Source: CAD feature listing. Evaluate the final solid. Frame: model axes, mm. A direction names the side the tool comes from. Round coordinates to 2 decimals unless told otherwise and drop trailing zeros. Write each loop counter-clockwise with the first axis right and the second up, starting at its lowest first coordinate (ties: lowest second). Pieces come first, ordered by that corner, then holes. Notation, with made-up numbers: (-21.5, 36) - (10.5, 36) arc R12 ccw to (10.5, 58) - close; hole circle Ø9 at (-20, 47). An arc over 180 degrees is marked (long way). Write item = value, one per line. Start each with the question number.
```python
from build123d import *

# Parameters (mm, degrees)
F1_DEPTH = 30
F2_W     = 40
F2_H     = 30
F3_DEPTH = 30
F5_DEPTH = 10
F7_D     = 20


with BuildPart() as f1:
    # F0 (on Front) → F1 (new body)
    with BuildSketch(Plane.XZ):
        Polygon((-1036.953415, 10), (-1046.953415, 0), (-966.953415, 0), (-976.953415, 10), align=None)
    extrude(amount=-F1_DEPTH)

    # F2 (on face) → F3 (join)
    with BuildSketch(Plane.XZ):
        with Locations((-1006.953415, 25)):
            Rectangle(F2_W, F2_H)
    extrude(amount=-F3_DEPTH)

    # F4 (on face) → F5 (join)
    with BuildSketch(Plane.XZ):
        with BuildLine():
            Line((-986.953415, 40), (-1026.953415, 40))
            ThreePointArc((-1026.953415, 40), (-1006.953415, 20), (-986.953415, 40))
        make_face()
    extrude(amount=F5_DEPTH)

    # F7 (through all)
    with Locations(Plane.XZ.offset(10)):
        with Locations((-1007.889872, 39.913703)):
            Hole(F7_D / 2)


solid = f1.part
```
(1) Ray query, L1, parallel to X at y = 28, z = 14; L2, parallel to Z at x = -979, y = 13; L3, parallel to X at y = 12, z = 33. Return the intervals inside material, ascending. Write a range as from..to.
(2) Reachability of faces 1 (the flat face through (-1022, 10, 40)), 2 (the flat face through (-1008, 15, 0)), 3 (the flat face through (-986.953, 15, 25)), 4 (the flat face through (-1032, 15, 10)), 5 (the cylindrical face through (-1007, -5, 20)) from +Z, -Z, +X, -X, +Y, -Y: full face, straight path, thin tool, end or side. Return the list, or none.
(3) Section C-C (z = 15.5). Return the cut outline in (x, y), plus the area to 3 significant figures.
(4) Section A-A (y = 25). Return the cut outline in (x, z).
(5) Section B-B (x = -1032). Return the cut outline in (y, z), plus the area to 3 significant figures.
(6) Pull-direction query (X, two-part tool) for faces 6 (the flat face through (-1008, 0, 11)), 7 (the flat face through (-971.883, 14.79, 4.93)), 8 (the cylindrical face through (-1007.669, 10.28, 29.916)), 9 (the flat face through (-1041.883, 14.79, 5.07)); classes: +X half, -X half, draft (parallel to the pull), parting line (faces both ways), or undercut.
(7) Contact query for flat-ended pins moving along their axis: P1, Ø11, axis at x = -1034.5, y = 9, coming from the +Z side; P2, Ø3, axis at x = -1006, z = 11, coming from the -Y side; P3, Ø1, axis at y = 25.5, z = 35, coming from the -X side; P4, Ø4, axis at y = -3, z = 7, coming from the +X side. Output: stop coordinate, or through.
Solution:
q1.L1 = -1026.95..-986.95
q1.L2 = 0..10
q1.L3 = -1026.95..-1015.11, -1000.66..-986.95
q2.face_1 = +Z, +X, -X, +Y, -Y
q2.face_2 = -Z, +X, -X, +Y, -Y
q2.face_3 = +Z, +X, +Y, -Y
q2.face_4 = +Z, -X, +Y, -Y
q2.face_5 = -Z, -Y
q3.outline = (-1026.95, 0) - (-986.95, 0) - (-986.95, 30) - (-1026.95, 30) - close
q3.area = 1,200 mm^2
q4.outline = (-1046.95, 0) - (-966.95, 0) - (-976.95, 10) - (-986.95, 10) - (-986.95, 40) - (-997.89, 40) arc R10 cw (long way) to (-1017.89, 40) - (-1026.95, 40) - (-1026.95, 10) - (-1036.95, 10) - close
q5.outline = (0, 0) - (30, 0) - (30, 10) - (0, 10) - close
q5.area = 300 mm^2
q6.face_6 = draft
q6.face_7 = +X half
q6.face_8 = undercut
q6.face_9 = -X half
q7.P1 = 10
q7.P2 = 0
q7.P3 = -1026.95
q7.P4 = through
